from build123d import *

# Parameters (mm, degrees)
BOSS_EXTRUDE1_START = -40.195413
SKETCH2_R           = 2.54
SKETCH2_W           = 117.366510392
SKETCH2_H           = 117.366510392
BOSS_EXTRUDE1_DEPTH = 40.195413
SKETCH8_W           = 123.716510392
SKETCH8_H           = 123.716510392
SKETCH8_W_2         = 117.366510392
SKETCH8_H_2         = 117.366510392
BOSS_EXTRUDE6_DEPTH = 38.1
SKETCH9_W           = 123.716510392
SKETCH9_H           = 123.716510392
BOSS_EXTRUDE7_DEPTH = 3.175
SKETCH11_W          = 203.085481381
SKETCH11_H          = 253.856851726
CUT_EXTRUDE3_DEPTH  = 35.56
SKETCH14_W          = 36.322
SKETCH14_H          = 15.24
SKETCH14_W_2        = 22.86
SKETCH14_H_2        = 22.86
CUT_EXTRUDE4_DEPTH  = 12.7


with BuildPart() as part:
    # Sketch2 → Boss-Extrude1 (new body)
    with BuildSketch(Plane.XY.offset(BOSS_EXTRUDE1_START)):
        with BuildLine():
            Line((1514.374964129, -9.898719074), (1513.372529957, -3.825593235))
            ThreePointArc((1513.372529957, -3.825593235), (1511.215570373, -0.017767746), (1507.107304519, 1.490264506))
            Line((1507.107304519, 1.490264506), (1506.145090959, 1.490264506))
            Line((1506.145090959, 1.490264506), (1505.274868714, 1.490264506))
            ThreePointArc((1505.274868714, 1.490264506), (1501.126253206, -0.052294453), (1498.993223216, -3.930526246))
            Line((1498.993223216, -3.930526246), (1498.110381295, -9.898719074))
            Line((1498.110381295, -9.898719074), (1494.935381295, -9.898719074))
            Line((1494.935381295, -9.898719074), (1444.2526074, -9.898719074))
            Line((1444.2526074, -9.898719074), (1444.2526074, -59.236149034))
            Line((1444.2526074, -59.236149034), (1444.2526074, -63.492872737))
            Line((1444.2526074, -63.492872737), (1438.179481561, -64.495306909))
            ThreePointArc((1438.179481561, -64.495306909), (1434.371656072, -66.652266493), (1432.86362382, -70.760532347))
            Line((1432.86362382, -70.760532347), (1432.86362382, -71.722745907))
            Line((1432.86362382, -71.722745907), (1432.86362382, -72.592968152))
            ThreePointArc((1432.86362382, -72.592968152), (1434.406182779, -76.74158366), (1438.284414571, -78.874613651))
            Line((1438.284414571, -78.874613651), (1444.2526074, -79.757455571))
            Line((1444.2526074, -79.757455571), (1444.2526074, -82.932455571))
            Line((1444.2526074, -82.932455571), (1444.2526074, -133.615229466))
            Line((1444.2526074, -133.615229466), (1493.590037359, -133.615229466))
            Line((1493.590037359, -133.615229466), (1497.846761063, -133.615229466))
            Line((1497.846761063, -133.615229466), (1498.849195235, -139.688355305))
            ThreePointArc((1498.849195235, -139.688355305), (1501.006154818, -143.496180794), (1505.114420673, -145.004213046))
            Line((1505.114420673, -145.004213046), (1506.076634233, -145.004213046))
            Line((1506.076634233, -145.004213046), (1506.946856478, -145.004213046))
            ThreePointArc((1506.946856478, -145.004213046), (1511.095471986, -143.461654087), (1513.228501976, -139.583422295))
            Line((1513.228501976, -139.583422295), (1514.111343897, -133.615229466))
            Line((1514.111343897, -133.615229466), (1517.286343897, -133.615229466))
            Line((1517.286343897, -133.615229466), (1567.969117792, -133.615229466))
            Line((1567.969117792, -133.615229466), (1567.969117792, -84.277799507))
            Line((1567.969117792, -84.277799507), (1567.969117792, -80.021075803))
            Line((1567.969117792, -80.021075803), (1574.042243631, -79.018641631))
            ThreePointArc((1574.042243631, -79.018641631), (1577.85006912, -76.861682048), (1579.358101372, -72.753416193))
            Line((1579.358101372, -72.753416193), (1579.358101372, -71.791202633))
            Line((1579.358101372, -71.791202633), (1579.358101372, -70.920980388))
            ThreePointArc((1579.358101372, -70.920980388), (1577.815542413, -66.77236488), (1573.93731062, -64.63933489))
            Line((1573.93731062, -64.63933489), (1567.969117792, -63.756492969))
            Line((1567.969117792, -63.756492969), (1567.969117792, -60.581492969))
            Line((1567.969117792, -60.581492969), (1567.969117792, -9.898719074))
            Line((1567.969117792, -9.898719074), (1518.631687833, -9.898719074))
            Line((1518.631687833, -9.898719074), (1514.374964129, -9.898719074))
        make_face()
        with Locations((1506.110862596, -138.695229466)):
            Circle(SKETCH2_R, mode=Mode.SUBTRACT)
        with Locations((1439.1726074, -71.75697427)):
            Circle(SKETCH2_R, mode=Mode.SUBTRACT)
        with Locations((1506.110862596, -71.75697427)):
            Rectangle(SKETCH2_W, SKETCH2_H, mode=Mode.SUBTRACT)
        with Locations((1506.110862596, -4.818719074)):
            Circle(SKETCH2_R, mode=Mode.SUBTRACT)
        with Locations((1573.049117792, -71.75697427)):
            Circle(SKETCH2_R, mode=Mode.SUBTRACT)
    extrude(amount=BOSS_EXTRUDE1_DEPTH)

    # Sketch8 → Boss-Extrude6 (add)
    with BuildSketch(Plane(origin=(0, 0, -40.195413), x_dir=(-1, 0, 0), z_dir=(0, 0, -1))):
        with Locations((-1506.110862596, -71.75697427)):
            Rectangle(SKETCH8_W, SKETCH8_H)
        with Locations((-1506.110862596, -71.75697427)):
            Rectangle(SKETCH8_W_2, SKETCH8_H_2, mode=Mode.SUBTRACT)
    extrude(amount=BOSS_EXTRUDE6_DEPTH)

    # Sketch9 → Boss-Extrude7 (add)
    with BuildSketch(Plane(origin=(0, 0, -78.295413), x_dir=(-1, 0, 0), z_dir=(0, 0, -1))):
        with Locations((-1506.110862596, -71.75697427)):
            Rectangle(SKETCH9_W, SKETCH9_H)
    extrude(amount=BOSS_EXTRUDE7_DEPTH)

    # Sketch11 → Cut-Extrude3 (cut)
    with BuildSketch(Plane.XY):
        with Locations((1484.541394478, -61.275179675)):
            Rectangle(SKETCH11_W, SKETCH11_H)
    extrude(amount=-CUT_EXTRUDE3_DEPTH, mode=Mode.SUBTRACT)

    # Sketch14 → Cut-Extrude4 (cut)
    with BuildSketch(Plane(origin=(1567.969117792, 0, 0), x_dir=(0, 0, -1), z_dir=(1, 0, 0))):
        with Locations((53.721, -113.66697427)):
            Rectangle(SKETCH14_W, SKETCH14_H)
        with Locations((54.102, -71.75697427)):
            Rectangle(SKETCH14_W_2, SKETCH14_H_2)
    extrude(amount=-CUT_EXTRUDE4_DEPTH, mode=Mode.SUBTRACT)


solid = part.part
Design review of the part built by this model. Coordinates are the model's own, in mm. A direction names the side the tool comes from. Give positions to 0.01 mm unless a question says otherwise; leave off trailing zeros. Order: outer loops, then holes, each group sorted by start corner. A loop starts at its lowest first (then second) coordinate and runs counter-clockwise, first axis right, second up.
1. Add section D-D, the plane z = -70. State the section outline as (x, y) points, then the cut area to 3 significant figures.
Solution:
outline: (1444.25, -133.62) - (1567.97, -133.62) - (1567.97, -121.29) - (1564.79, -121.29) - (1564.79, -130.44) - (1447.43, -130.44) - (1447.43, -13.07) - (1564.79, -13.07) - (1564.79, -106.05) - (1567.97, -106.05) - (1567.97, -9.9) - (1444.25, -9.9) - close
area: 1,480 mm2
2. For pin 1 Ø3.5 at (x, z) = (1567, -51) entering from -Y; pin 2 Ø6 at (y, z) = (-112, -47.5) entering from -X; pin 3 Ø12 at (y, z) = (-116.5, -41) entering from +X; pin 4 Ø6 at (x, y) = (1439.17, -71.76) entering from +Z, all flat-tipped, find the tip position at first contact; note any pin that passes through.
Solution:
pin 1: stops at y = -133.62
pin 2: stops at x = 1444.25
pin 3: stops at x = 1567.97
pin 4: stops at z = -35.56
3. Add section A-A, the plane z = -46. State the section outline as (x, y) points.
Solution:
outline: (1444.25, -133.62) - (1567.97, -133.62) - (1567.97, -121.29) - (1564.79, -121.29) - (1564.79, -130.44) - (1447.43, -130.44) - (1447.43, -13.07) - (1564.79, -13.07) - (1564.79, -60.33) - (1567.97, -60.33) - (1567.97, -9.9) - (1444.25, -9.9) - close; (1564.79, -106.05) - (1567.97, -106.05) - (1567.97, -83.19) - (1564.79, -83.19) - close
4. Mouldability with a two-part tool opening along Y and no side actions: class faces 4 (the cylindrical face through (1511.05, -143.5, -37.91)), 5 (the flat face through (1507, -13.074, -57)), 6 (the flat face through (1570.995, -64.204, -37.91)) as +Y half, -Y half, draft (parallel to the pull), parting line (faces both ways), or undercut.
Solution:
face 4: -Y half
face 5: undercut
face 6: +Y half
5. Add section B-B, the plane y = -42. State the section outline as (x, z) points.
Solution:
outline: (1444.25, -81.47) - (1567.97, -81.47) - (1567.97, -35.56) - (1564.79, -35.56) - (1564.79, -78.3) - (1447.43, -78.3) - (1447.43, -35.56) - (1444.25, -35.56) - close
6. To check wall thickness, follow L1, parallel to Y at x = 1566.5, z = -43; L2, parallel to X at y = -65, z = -72; L3, parallel to Y at x = 1542, z = -50. State the ranges of each line that lie inside material, in increasing order.
Solution:
L1: y = -133.62 to -121.29, -106.05 to -83.19, -60.33 to -9.9
L2: x = 1444.25 to 1447.43, 1564.79 to 1567.97
L3: y = -133.62 to -130.44, -13.07 to -9.9
7. Tool access review of faces 1 (the flat face through (1513.664, -136.641, -37.91)), 2 (the flat face through (1564.794, -60, -57)), 3 (the flat face through (1575, -74, -40.195)): name each direction out of +Z, -Z, +X, -X, +Y, -Y from which nothing blocks a thin tool from reaching the whole face with its end or side.
Solution:
face 1: +Z, -Z, +X, -Y
face 2: +Z
face 3: -Z, +X, +Y, -Y
8. Add section C-C, the plane x = 1551.5. State the section outline as (y, z) points, then the cut area to 3 significant figures.
Solution:
outline: (-133.62, -81.47) - (-9.9, -81.47) - (-9.9, -35.56) - (-13.07, -35.56) - (-13.07, -78.3) - (-130.44, -78.3) - (-130.44, -35.56) - (-133.62, -35.56) - close
area: 664 mm2
